For this review, take the finished solid that the model builds, in its own axes (mm). Round coordinates to 2 decimals unless told otherwise and drop trailing zeros. Order: outer loops, then holes, each group sorted by start corner. A loop starts at its lowest first (then second) coordinate and runs counter-clockwise, first axis right, second up. Notation, with made-up numbers: (69, 6.5) -> (87, 6.5) arc R23 cw to (87, 31.5) -> close; hole circle Ø2 at (24, 66.5). An arc over 180 degrees is marked (long way). Use a Markdown table: item, result. Add a question column.
1) Clearance check with flat-ended pins moving along their axes: P1, Ø4, axis at y = -30, z = -25, coming from the -X side; P2, Ø1.9, axis at x = -1.5, y = 69, coming from the -Z side; P3, Ø1.9, axis at x = -3.5, z = 15, coming from the +Y side (3 decimals). State where each tip first meets the part, or that it passes through.
2) Wall thickness on line 1 along Y through (x, z) = (-0.25, -71) (3 decimals); line 2 along X through (y, z) = (-230, 80): over which ranges is each line inside the solid? List them lowest first. Write a range as [from, to].
3) Consider section B-B (y = -19.5). State the section outline as (x, z) points.
4) Consider section C-C (z = -87.5). State the section outline as (x, y) points.
5) Consider section A-A (z = 9.5). State the section outline as (x, y) points (3 decimals), plus the area to 3 significant figures.
```python
from build123d import *

# Parameters (mm, degrees)
F0_W     = 508
F0_H     = 203.2
F1_DEPTH = 19.05
F2_W     = 12.7
F2_H     = 101.6
F2_H_2   = 76.2
F3_DEPTH = 6.35


with BuildPart() as f1:
    # F0 (on Right) → F1 (new body)
    with BuildSketch(Plane.YZ):
        Rectangle(F0_W, F0_H)
    extrude(amount=F1_DEPTH)

    # F2 (on face) → F3 (join)
    with BuildSketch(Plane(origin=(0, 0, 0), x_dir=(0, -1, 0), z_dir=(-1, 0, 0))):
        with Locations((-66.675, 50.8)):
            Rectangle(F2_W, F2_H)
        with Locations((-66.675, -38.1)):
            Rectangle(F2_W, F2_H_2)
        with Locations((-34.925, -38.1)):
            Rectangle(F2_W, F2_H_2)
        with Locations((-34.925, 50.8)):
            Rectangle(F2_W, F2_H)
    extrude(amount=F3_DEPTH)


solid = f1.part
```
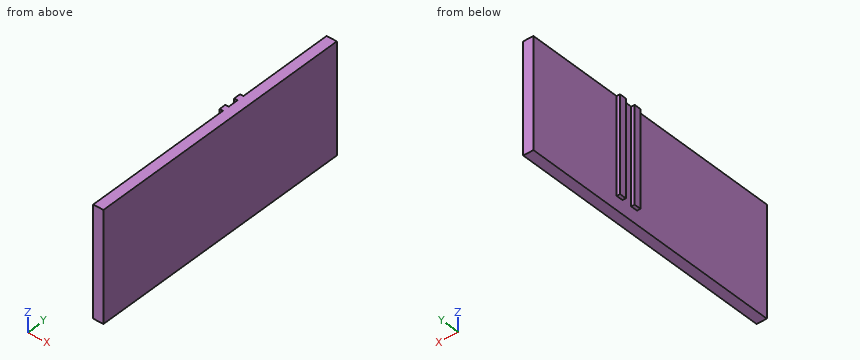
Results list:
| question | item | result |
|---|---|---|
| 1 | P1 | x = 0 |
| 1 | P2 | z = -76.2 |
| 1 | P3 | y = 73.025 |
| 2 | line 1 | [28.575, 41.275], [60.325, 73.025] |
| 2 | line 2 | [0, 19.05] |
| 3 | outline | (0, -101.6) -> (19.05, -101.6) -> (19.05, 101.6) -> (0, 101.6) -> close |
| 4 | outline | (0, -254) -> (19.05, -254) -> (19.05, 254) -> (0, 254) -> close |
| 5 | outline | (-6.35, 28.575) -> (0, 28.575) -> (0, -254) -> (19.05, -254) -> (19.05, 254) -> (0, 254) -> (0, 73.025) -> (-6.35, 73.025) -> (-6.35, 60.325) -> (0, 60.325) -> (0, 41.275) -> (-6.35, 41.275) -> close |
| 5 | area | 9,840 mm2 |
